```python
from build123d import *

# Parameters (mm, degrees)
SKETCH1_W                      = 65
SKETCH1_H                      = 32
EXTRUDE1_DEPTH                 = 6.35
CBORE_FOR_M3_SHCS2_D           = 3.4
CBORE_FOR_M3_SHCS2_CBORE_D     = 6.5
CBORE_FOR_M3_SHCS2_CBORE_DEPTH = 4
LPATTERN1_COUNT                = 2
LPATTERN1_PITCH                = 25
LPATTERN1_COUNT_DIR2           = 2
LPATTERN1_PITCH_DIR2           = 25
LPATTERN2_COUNT                = 2
LPATTERN2_PITCH                = 58
LPATTERN2_COUNT_DIR2           = 2
LPATTERN2_PITCH_DIR2           = 25


with BuildPart() as part:
    # Sketch1 → Extrude1 (new body)
    with BuildSketch(Plane(origin=(0, 0, 0), x_dir=(1, 0, 0), z_dir=(0, 1, 0))):
        Rectangle(SKETCH1_W, SKETCH1_H)
    extrude(amount=EXTRUDE1_DEPTH)

    # CBORE for M3 SHCS2 (through all)
    with Locations(Plane(origin=(-12.5, 6.35, -12.5), x_dir=(0, 0, 1), z_dir=(0, 1, 0))):
        with Locations((0, 0)):
            cbore_for_m3_shcs2 = CounterBoreHole(CBORE_FOR_M3_SHCS2_D / 2, CBORE_FOR_M3_SHCS2_CBORE_D / 2, CBORE_FOR_M3_SHCS2_CBORE_DEPTH)

    # LPattern1: CBORE for M3 SHCS2 2 × 2
    with Locations(*[(i * LPATTERN1_PITCH, 0, j * LPATTERN1_PITCH_DIR2) for i in range(LPATTERN1_COUNT) for j in range(LPATTERN1_COUNT_DIR2) if (i, j) != (0, 0)]):
        add(cbore_for_m3_shcs2, mode=Mode.SUBTRACT)

    # Sketch5 → M4x0.7 Tapped Hole1 (revolve, cut)
    with BuildSketch(Plane(origin=(-29, 6.35, -12.5), x_dir=(0, 0, 1), z_dir=(1, 0, 0))):
        Polygon((0, 0), (0, 12.491420021), (1.65, 11.5), (1.65, 0), align=None)
    m4x0_7_tapped_hole1 = revolve(axis=Axis((-29, 12.7, -12.5), (0, -1, 0)), mode=Mode.SUBTRACT)

    # LPattern2: M4x0.7 Tapped Hole1 2 × 2
    with Locations(*[(i * LPATTERN2_PITCH, 0, j * LPATTERN2_PITCH_DIR2) for i in range(LPATTERN2_COUNT) for j in range(LPATTERN2_COUNT_DIR2) if (i, j) != (0, 0)]):
        add(m4x0_7_tapped_hole1, mode=Mode.SUBTRACT)


solid = part.part
```
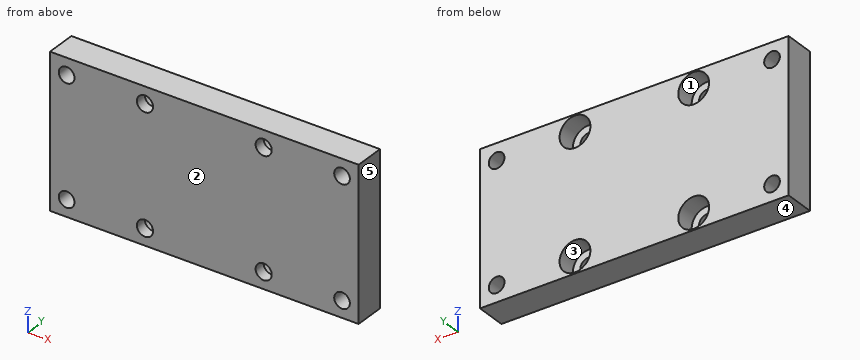
Verification items for the finished model (mm, model axes). Face numbers are marked on the shaded views. A direction names the side the tool comes from. Round coordinates to 2 decimals unless told otherwise and drop trailing zeros. Loops run counter-clockwise (first coordinate to the right, second up) from the corner with the lowest first, then second, coordinate; pieces in that order, holes last. Notation, with made-up numbers: (49, 58.5) -> (74, 58.5) arc R20 ccw to (74, 88.5) -> close; hole circle Ø4 at (23, 84.25). An arc over 180 degrees is marked (long way). Answer as a JSON object with one key per item and string values.
Q1. Draft check along X on the marked faces 3, 4 and 5. Enter one of: pulls with the +X half, pulls with the -X half, needs draft (parallel to the pull), parting line crosses it, or undercut.
Data:
{"face 3": "undercut", "face 4": "needs draft", "face 5": "pulls with the +X half"}
Q2. Scan lines: line 1 (X direction, y = 0.5, z = -12.5); line 2 (X direction, y = 4.55, z = -12.5); line 3 (Y direction, x = -14.5, z = -11.5). Record each from-to range of solid material in increasing order. Write a range as from..to.
Data:
{"line 1": "x = -32.5..-30.65, -27.35..-14.2, -10.8..10.8, 14.2..27.35, 30.65..32.5", "line 2": "x = -32.5..-30.65, -27.35..-15.75, -9.25..9.25, 15.75..27.35, 30.65..32.5", "line 3": "y = 0..2.35"}
Q3. Section check B-B (y = 4.75). State how many separate pieces and enclosed holes the cut face has, then the cut area to 3 significant figures.
Data:
{"separate pieces": "1", "enclosed holes": "8", "area": "1,910 mm2"}
Q4. Access from +Z, -Z, +X, -X, +Y, -Y to the whole of each face (thin tool, end or side, straight path). Record for the marked faces 1 and 2.
Data:
{"face 1": "+Y", "face 2": "+Z, -Z, +X, -X, -Y"}
Q5. Section check D-D (x = -29). Record the boundary of the cut face in (y, z), then the cut area to 3 significant figures.
Data:
{"outline": "(0, -16) -> (6.35, -16) -> (6.35, -14.15) -> (0, -14.15) -> close; (0, -10.85) -> (6.35, -10.85) -> (6.35, 10.85) -> (0, 10.85) -> close; (0, 14.15) -> (6.35, 14.15) -> (6.35, 16) -> (0, 16) -> close", "area": "161 mm2"}
Q6. Go/stop test with a flat-tipped pin: P1, Ø3, axis at x = -11, z = -13, coming from the +Y side. Record where the tip stops, or that it passes through.
Data:
{"P1": "stops at y = 2.35"}
Q7. Section check C-C (x = -13.5). Record the boundary of the cut face in (y, z).
Data:
{"outline": "(0, -16) -> (6.35, -16) -> (6.35, -15.59) -> (2.35, -15.59) -> (2.35, -13.87) -> (0, -13.87) -> close; (0, -11.13) -> (2.35, -11.13) -> (2.35, -9.41) -> (6.35, -9.41) -> (6.35, 9.41) -> (2.35, 9.41) -> (2.35, 11.13) -> (0, 11.13) -> close; (0, 13.87) -> (2.35, 13.87) -> (2.35, 15.59) -> (6.35, 15.59) -> (6.35, 16) -> (0, 16) -> close"}
Q8. Section check A-A (z = -12.5). Record the boundary of the cut face in (x, y), then the cut area to 3 significant figures.
Data:
{"outline": "(-32.5, 0) -> (-30.65, 0) -> (-30.65, 6.35) -> (-32.5, 6.35) -> close; (-27.35, 0) -> (-14.2, 0) -> (-14.2, 2.35) -> (-15.75, 2.35) -> (-15.75, 6.35) -> (-27.35, 6.35) -> close; (-10.8, 0) -> (10.8, 0) -> (10.8, 2.35) -> (9.25, 2.35) -> (9.25, 6.35) -> (-9.25, 6.35) -> (-9.25, 2.35) -> (-10.8, 2.35) -> close; (14.2, 0) -> (27.35, 0) -> (27.35, 6.35) -> (15.75, 6.35) -> (15.75, 2.35) -> (14.2, 2.35) -> close; (30.65, 0) -> (32.5, 0) -> (32.5, 6.35) -> (30.65, 6.35) -> close", "area": "303 mm2"}
